Design review of the part built by this model. Coordinates are the model's own, in mm. Face numbers are marked on the shaded views. Coordinates: 2 decimals unless noted, no trailing zeros. Loops run counter-clockwise (first coordinate to the right, second up) from the corner with the lowest first, then second, coordinate; pieces in that order, holes last.
Q1. Wall thickness on probe 1 along Z at (x, y) = (11.75, 0); probe 2 along Y at (x, z) = (11.5, -21.5); probe 3 along Z at (x, y) = (7.25, 0): over which ranges is each line inside the solid? List them lowest first.
Q2. Add section C-C on z = 267. Give the boundary of the cut face in (x, y).
Q3. Add section B-B on z = 0. Give the boundary of the cut face in (x, y) (3 decimals), and give its area (3 significant figures).
Q4. Draft analysis for pull direction X (two halves, no side actions). For the marked faces 1 and 2, state which applies: released by +X, released by -X, zero draft, split by the parting line, or undercut.
Q5. Add section A-A on y = 0. Give the boundary of the cut face in (x, z) (3 decimals).
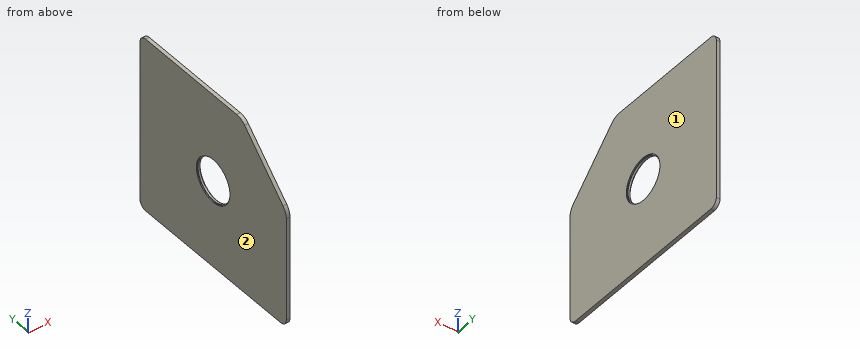
```python
from build123d import *

# Parameters (mm, degrees)
F1_DEPTH = 12.7
F2_R     = 72.517
F3_DEPTH = 12.701
F4_R     = 75.692
F5_DEPTH = 3.175
F6_R     = 75.692
F7_DEPTH = 3.175


with BuildPart() as f1:
    # F0 (on Right) → F1 (new body)
    with BuildSketch(Plane.YZ):
        with BuildLine():
            ThreePointArc((330.2, 279.4), (322.760512, 297.360512), (304.8, 304.8))
            Line((304.8, 304.8), (-105.957951, 304.8))
            ThreePointArc((-105.957951, 304.8), (-125.398269, 300.93308), (-141.878976, 289.921024))
            Line((-141.878976, 289.921024), (-315.321024, 116.478976))
            ThreePointArc((-315.321024, 116.478976), (-326.33308, 99.998269), (-330.2, 80.557951))
            Line((-330.2, 80.557951), (-330.2, -279.4))
            ThreePointArc((-330.2, -279.4), (-322.760512, -297.360512), (-304.8, -304.8))
            Line((-304.8, -304.8), (304.8, -304.8))
            ThreePointArc((304.8, -304.8), (322.760512, -297.360512), (330.2, -279.4))
            Line((330.2, -279.4), (330.2, 279.4))
        make_face()
    extrude(amount=F1_DEPTH)

    # F2 (on face) → F3 (cut, through all)
    with BuildSketch(Plane.YZ.offset(12.7)):
        Circle(F2_R)
    extrude(amount=-F3_DEPTH, mode=Mode.SUBTRACT)

    # F4 (on face) → F5 (cut)
    with BuildSketch(Plane.YZ.offset(12.7)):
        Circle(F4_R)
    extrude(amount=-F5_DEPTH, mode=Mode.SUBTRACT)

    # F6 (on face) → F7 (cut)
    with BuildSketch(Plane(origin=(0, 0, 0), x_dir=(0, -1, 0), z_dir=(-1, 0, 0))):
        Circle(F6_R)
    extrude(amount=-F7_DEPTH, mode=Mode.SUBTRACT)


solid = f1.part
```
Entries:
1. probe 1: z = -304.8 to -75.69, 75.69 to 304.8
1. probe 2: y = -330.2 to -72.57, 72.57 to 330.2
1. probe 3: z = -304.8 to -72.52, 72.52 to 304.8
2. outline: (0, -164.8) - (12.7, -164.8) - (12.7, 330.2) - (0, 330.2) - close
3. outline: (0, -330.2) - (12.7, -330.2) - (12.7, -75.692) - (9.525, -75.692) - (9.525, -72.517) - (3.175, -72.517) - (3.175, -75.692) - (0, -75.692) - close; (0, 75.692) - (3.175, 75.692) - (3.175, 72.517) - (9.525, 72.517) - (9.525, 75.692) - (12.7, 75.692) - (12.7, 330.2) - (0, 330.2) - close
3. area: 6,500 mm2
4. face 1: released by +X
4. face 2: released by -X
5. outline: (0, -304.8) - (12.7, -304.8) - (12.7, -75.692) - (9.525, -75.692) - (9.525, -72.517) - (3.175, -72.517) - (3.175, -75.692) - (0, -75.692) - close; (0, 75.692) - (3.175, 75.692) - (3.175, 72.517) - (9.525, 72.517) - (9.525, 75.692) - (12.7, 75.692) - (12.7, 304.8) - (0, 304.8) - close
